```python
from build123d import *

# Parameters (mm, degrees)
SKETCH1_W           = 79
SKETCH1_H           = 28
BOSS_EXTRUDE1_DEPTH = 60
CUT_EXTRUDE1_DEPTH  = 46
SKETCH3_W           = 25.74
SKETCH3_H           = 3
CUT_EXTRUDE2_DEPTH  = 26
CUT_EXTRUDE3_DEPTH  = 26
FILLET1_R           = 1.55
FILLET2_R           = 2


with BuildPart() as part:
    # Sketch1 → Boss-Extrude1 (new body)
    with BuildSketch(Plane.XY):
        with Locations((39.5, 14)):
            Rectangle(SKETCH1_W, SKETCH1_H)
    extrude(amount=BOSS_EXTRUDE1_DEPTH)

    # Sketch2 → Cut-Extrude1 (cut)
    with BuildSketch(Plane.XY.offset(60)):
        Polygon((3.45, 26.05), (75.6, 26.05), (77.15, 26.05), (77.15, 24.45), (75.55, 24.45), (75.55, 1.95), (3.45, 1.95), (3.45, 24.45), (1.85, 24.45), (1.85, 26.05), align=None)
    extrude(amount=-CUT_EXTRUDE1_DEPTH, mode=Mode.SUBTRACT)

    # Sketch3 → Cut-Extrude2 (cut)
    with BuildSketch(Plane.XY.offset(14)):
        with Locations((61.13, 5)):
            Rectangle(SKETCH3_W, SKETCH3_H)
    extrude(amount=-CUT_EXTRUDE2_DEPTH, mode=Mode.SUBTRACT)

    # Sketch4 → Cut-Extrude3 (cut)
    with BuildSketch(Plane.XY.offset(14)):
        Polygon((6.45, 24.05), (72.55, 24.05), (72.55, 8.5), (46.26, 8.5), (46.26, 3.95), (6.45, 3.95), align=None)
    extrude(amount=-CUT_EXTRUDE3_DEPTH, mode=Mode.SUBTRACT)

    # Fillet1
    fillet1_edges = [part.edges().sort_by_distance(p)[0] for p in [
        (75.55, 1.95, 37),
        (3.45, 1.95, 37),
    ]]
    fillet(fillet1_edges, radius=FILLET1_R)

    # Fillet2
    fillet2_edges = [part.edges().sort_by_distance(p)[0] for p in [
        (6.45, 3.95, 7),
        (6.45, 24.05, 7),
        (72.55, 24.05, 7),
        (72.55, 8.5, 7),
        (46.26, 8.5, 7),
        (46.26, 3.95, 7),
    ]]
    fillet(fillet2_edges, radius=FILLET2_R)


solid = part.part
```
Could you check a few things on this model? Use its own coordinates, in mm. A direction names the side the tool comes from. Round coordinates to 2 decimals unless told otherwise and drop trailing zeros. Write each loop counter-clockwise with the first axis right and the second up, starting at its lowest first coordinate (ties: lowest second). Pieces come first, ordered by that corner, then holes. Notation, with made-up numbers: M 56,13 L 82,13 A5 ccw 82,19 Z; hole C 84.5,-32.75 d1. An arc over 180 degrees is marked long. Answer in a Markdown table with one row per item. Add a question column.
Q1. If we mould it in two halves opening along Y, with no side actions, what happens to faces 3 (the cylindrical face through (7.05, 23.48, 6.9)), 4 (the flat face through (79, 14, 30))? For each: +Y half, -Y half, draft (parallel to the pull), parting line (faces both ways), or undercut.
Q2. Imagine slicing it at A-A (x = 32). Please give me the cut outline in (y, z).
Q3. If I drill on line 1 (X direction, y = 16.75, z = 15.5); line 2 (X direction, y = 17.5, z = 9); line 3 (Y direction, x = 69.5, z = 48), over which ranges is the centre line in solid material (lowest first)? Write a range as from..to.
Q4. Imagine slicing it at D-D (x = 66). Please give me the cut outline in (y, z), then the cut area to 3 significant figures.
Q5. Imagine slicing it at C-C (y = 19.75). Please give me the cut outline in (x, z), then the cut area to 3 significant figures.
Q6. On a 3-axis mill with a long thin cutter (end or side, diameter ignored), from which of +Z, -Z, +X, -X, +Y, -Y can I reach the whole of each face in a straight line? I mean faces 1 (the flat face through (40, 1.95, 37)), 2 (the cylindrical face through (71.98, 9.1, 6.9)). Say none if no direction works.
Q7. Imagine slicing it at B-B (z = 27). Please give me the cut outline in (x, y), then the cut area to 3 significant figures.
Values:
| question | item | result |
|---|---|---|
| 1 | face 3 | undercut |
| 1 | face 4 | draft |
| 2 | outline | M 0,0 L 3.95,0 L 3.95,14 L 1.95,14 L 1.95,60 L 0,60 Z; M 24.05,0 L 28,0 L 28,60 L 26.05,60 L 26.05,14 L 24.05,14 Z |
| 3 | line 1 | 0..3.45, 75.55..79 |
| 3 | line 2 | 0..6.45, 72.55..79 |
| 3 | line 3 | 0..1.95, 26.05..28 |
| 4 | outline | M 0,0 L 3.5,0 L 3.5,14 L 1.95,14 L 1.95,60 L 0,60 Z; M 6.5,0 L 8.5,0 L 8.5,14 L 6.5,14 Z; M 24.05,0 L 28,0 L 28,60 L 26.05,60 L 26.05,14 L 24.05,14 Z |
| 4 | area | 312 mm^2 |
| 5 | outline | M 0,0 L 6.45,0 L 6.45,14 L 3.45,14 L 3.45,60 L 0,60 Z; M 72.55,0 L 79,0 L 79,60 L 75.55,60 L 75.55,14 L 72.55,14 Z |
| 5 | area | 498 mm^2 |
| 6 | face 1 | +Z |
| 6 | face 2 | +Z, -Z |
| 7 | outline | M 0,0 L 79,0 L 79,28 L 0,28 Z; hole M 1.85,24.45 L 3.45,24.45 L 3.45,3.5 A1.55 ccw 5,1.95 L 74,1.95 A1.55 ccw 75.55,3.5 L 75.55,24.45 L 77.15,24.45 L 77.15,26.05 L 1.85,26.05 Z |
| 7 | area | 470 mm^2 |
